Drawing for the job (mm, zero at the part's lowest x, y, z). Coordinates: 2 decimals unless noted, no trailing zeros. Order: outer loops, then holes, each group sorted by start corner. A loop starts at its lowest first (then second) coordinate and runs counter-clockwise, first axis right, second up.
1) Mould opens along X. For the marked faces 1, 2 and 3 say: +X half, -X half, draft (parallel to the pull), parting line (faces both ways), or undercut.
2) Pin check, flat tips, straight feed: pin 1 Ø0.9 at (y, z) = (5, 15) entering from -X; pin 2 Ø1.4 at (x, y) = (19, 3) entering from +Z. Stop position of each tip, or through.
3) Cut at D-D (z = 4). List the corners of the cut face in (x, y) (1 decimal), and give its area (3 significant figures).
4) Wall check: L1, parallel to Y at x = 55.88, z = 13; L2, parallel to X at y = 2.75, z = 6.35 (3 decimals); L3, parallel to Z at x = 6.35, y = 2.75 (3 decimals). Give the ranges that are in metal, low to high.
5) Cut at C-C (x = 20.32). List the corners of the cut face in (y, z), and give its area (3 significant figures).
6) Cut at A-A (z = 7.75). List the corners of the cut face in (x, y), and give its area (3 significant figures).
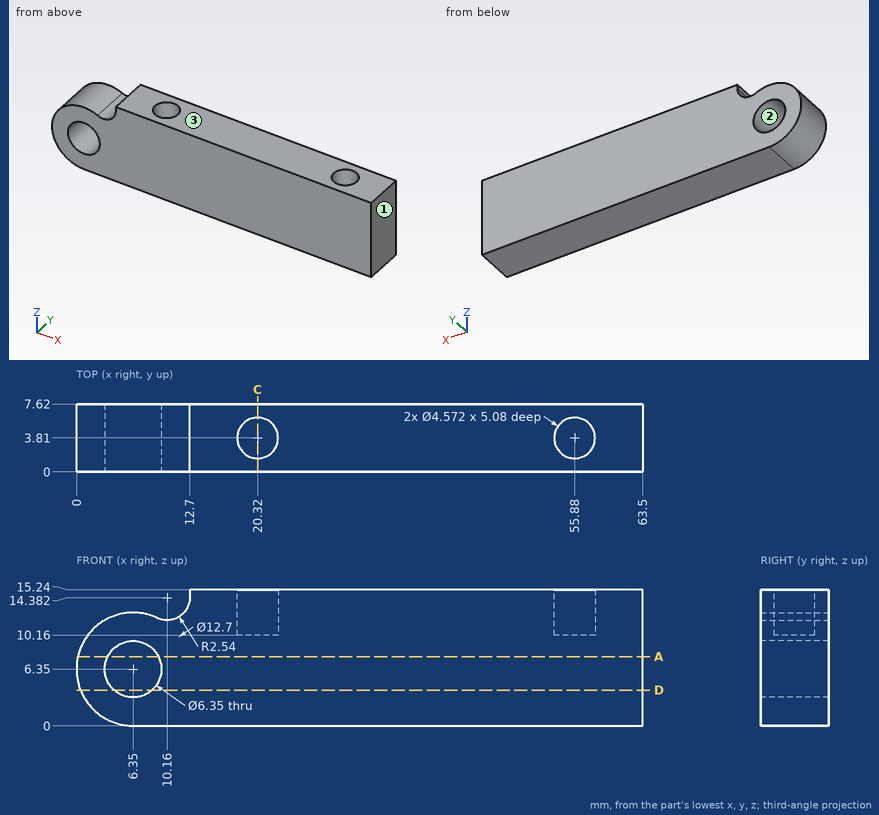
Geometry check:
1. face 1: +X half
1. face 2: undercut
1. face 3: draft
2. pin 1: stops at x = 12.7
2. pin 2: stops at z = 10.16
3. outline: (0.5, 0) - (4.2, 0) - (4.2, 7.6) - (0.5, 7.6) - close; (8.5, 0) - (63.5, 0) - (63.5, 7.6) - (8.5, 7.6) - close
3. area: 448 mm2
4. L1: y = 0 to 1.52, 6.1 to 7.62
4. L2: x = 0 to 3.175, 9.525 to 63.5
4. L3: z = 0 to 3.175, 9.525 to 12.7
5. outline: (0, 0) - (7.62, 0) - (7.62, 15.24) - (6.1, 15.24) - (6.1, 10.16) - (1.52, 10.16) - (1.52, 15.24) - (0, 15.24) - close
5. area: 92.9 mm2
6. outline: (0.16, 0) - (3.5, 0) - (3.5, 7.62) - (0.16, 7.62) - close; (9.2, 0) - (63.5, 0) - (63.5, 7.62) - (9.2, 7.62) - close
6. area: 439 mm2
